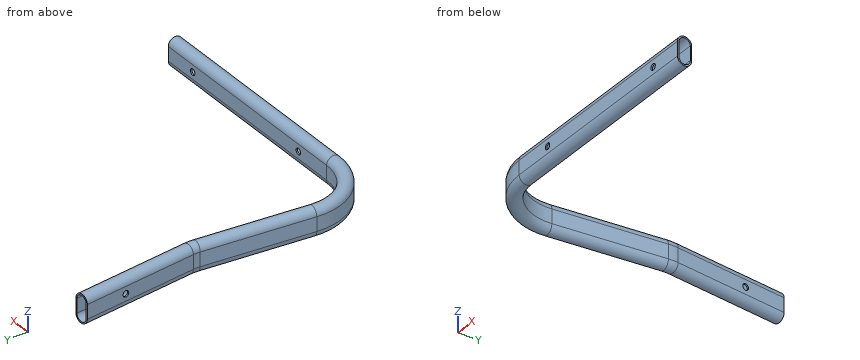
from build123d import *

# Parameters (mm, degrees)
SKETCH_3_R          = 3.3
CUT_EXTRUDE_1_DEPTH = 435.163655166
SKETCH_4_R          = 3.3
CUT_EXTRUDE_2_DEPTH = 432.316912752


with BuildPart() as part:
    # По траектории1: sweep along a path in Эскиз1
    with BuildLine(Plane.XY) as sweep_1_path:
        Line((0, 0), (-240, 0))
        ThreePointArc((-240, 0), (-287.923026893, 21.086636505), (-304.752655376, 70.665123279))
        Line((-304.752655376, 70.665123279), (-294.57908638, 186.949549004))
        ThreePointArc((-294.57908638, 186.949549004), (-294.451231483, 190.610834225), (-294.706785506, 194.265427019))
        Line((-294.706785506, 194.265427019), (-309.776696157, 317))
    # Эскиз2 → По траектории1 (sweep)
    with BuildSketch(Plane(origin=(0, 0, 0), x_dir=(0, 0, -1), z_dir=(1, 0, 0))):
        with BuildLine():
            Line((-7.5, 15), (7.5, 15))
            ThreePointArc((7.5, 15), (15, 7.5), (7.5, 0))
            Line((7.5, 0), (-7.5, 0))
            ThreePointArc((-7.5, 0), (-15, 7.5), (-7.5, 15))
        make_face()
        with BuildLine():
            Line((-7.5, 13.5), (7.5, 13.5))
            ThreePointArc((7.5, 13.5), (13.5, 7.5), (7.5, 1.5))
            Line((7.5, 1.5), (-7.5, 1.5))
            ThreePointArc((-7.5, 1.5), (-13.5, 7.5), (-7.5, 13.5))
        make_face(mode=Mode.SUBTRACT)
    sweep(path=sweep_1_path.line)

    # Эскиз3 → Вырез-Вытянуть1 (cut, through all)
    with BuildSketch(Plane(origin=(0, 15, 0), x_dir=(1, 0, 0), z_dir=(0, 1, 0))):
        with Locations(Location((-197, 0, 0), (0, 0, 180))):
            Circle(SKETCH_3_R)
        with Locations(Location((-37, 0, 0), (0, 0, 180))):
            Circle(SKETCH_3_R)
    extrude(amount=-CUT_EXTRUDE_1_DEPTH, mode=Mode.SUBTRACT)

    # Эскиз4 → Вырез-Вытянуть2 (cut, through all)
    with BuildSketch(Plane(origin=(-251.943037542, -30.934715237, 0), x_dir=(0, 0, -1), z_dir=(0.9925461516413225, 0.12186934340514467, 0))):
        with Locations(Location((0, 307.389412633, 0), (0, 0, 90))):
            Circle(SKETCH_4_R)
    extrude(amount=-CUT_EXTRUDE_2_DEPTH, mode=Mode.SUBTRACT)


solid = part.part
Could you check a few things on this model? Use its own coordinates, in mm. Give positions to 0.01 mm unless a question says otherwise; leave off trailing zeros. Order: outer loops, then holes, each group sorted by start corner. A loop starts at its lowest first (then second) coordinate and runs counter-clockwise, first axis right, second up. Notation, with made-up numbers: (40, -21) -> (74, -21) arc R16 cw to (74, 3) -> close; hole circle Ø11 at (-17, 13.25). An arc over 180 degrees is marked (long way). Answer in a Markdown table with one row per item. Add a question column.
Item 1: Please list where these lines run through material, in increasing order: probe 1 along Y at (x, z) = (-87, 0); probe 2 along Z at (x, y) = (-37, 14); probe 3 along Y at (x, z) = (-246, -11).
Item 2: Imagine slicing it at A-A (x = -188). List the corners of the cut face in (y, z) for me.
Item 3: I'm going to push flat-ended pins straight in: P1, Ø4.5, axis at x = -66, z = 2, coming from the +Y side; P2, Ø1, axis at y = 44, z = 2, coming from the +X side; P3, Ø10, axis at y = 91, z = 2.5, coming from the -X side. Where does each tip first touch, or does it pass through?
Result:
| question | item | result |
|---|---|---|
| 1 | probe 1 | 0 to 1.5, 13.5 to 15 |
| 1 | probe 2 | -11.24 to -3.3, 3.3 to 11.24 |
| 1 | probe 3 | 1.15 to 2.92, 12.72 to 14.49 |
| 2 | outline | (0, -7.5) arc R7.5 ccw to (15, -7.5) -> (15, 7.5) arc R7.5 ccw to (0, 7.5) -> close; hole (1.5, -7.5) arc R6 ccw to (13.5, -7.5) -> (13.5, 7.5) arc R6 ccw to (1.5, 7.5) -> close |
| 3 | P1 | y = 15 |
| 3 | P2 | x = -285.14 |
| 3 | P3 | x = -303.41 |
